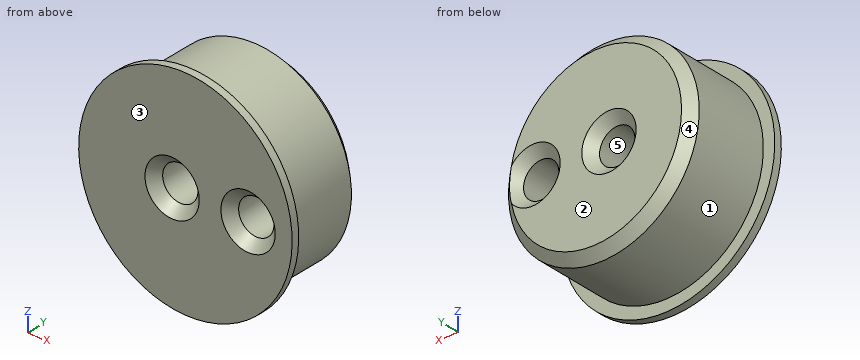
```python
from build123d import *
from build123d.topology import SkipClean

# Parameters (mm, degrees)
SKETCH_1_R      = 5.02
SKETCH_1_R_2    = 0.93
EXTRUDE_1_DEPTH = 4.4
EXTRUDE_START   = 0.4
SKETCH_3_R      = 5.62
SKETCH_3_R_2    = 0.93
EXTRUDE_2_DEPTH = 0.4
CHAMFER_1_SIZE  = 0.5


with BuildPart() as part:
    # 草图1 → 凸台-拉伸1 (new body)
    with BuildSketch(Plane(origin=(0, 0, 0), x_dir=(1, 0, 0), z_dir=(0, 1, 0))):
        with Locations(Location((0, 0, 0), (0, 0, 270))):
            Circle(SKETCH_1_R)
        with Locations(Location((3.3, 0, 0), (0, 0, 270))):
            Circle(SKETCH_1_R_2, mode=Mode.SUBTRACT)
        with Locations(Location((-0.7, 0, 0), (0, 0, 90))):
            Circle(SKETCH_1_R_2, mode=Mode.SUBTRACT)
    extrude(amount=EXTRUDE_1_DEPTH)

    # 草图3 → 凸台-拉伸2 (add)
    with SkipClean():  # the faces are left unmerged after this step: merging them gives an invalid solid
        with BuildSketch(Plane.XZ.offset(EXTRUDE_START)):
            with Locations(Location((0, 0, 0), (0, 0, 270))):
                Circle(SKETCH_3_R)
            with Locations(Location((3.3, 0, 0), (0, 0, 270))):
                Circle(SKETCH_3_R_2, mode=Mode.SUBTRACT)
            with Locations(Location((-0.7, 0, 0), (0, 0, 270))):
                Circle(SKETCH_3_R_2, mode=Mode.SUBTRACT)
        extrude(amount=-EXTRUDE_2_DEPTH)

    # 倒角1
    # the kernel refuses this chamfer: 0.5 mm, written as the material it takes off along each edge
    with BuildSketch(Plane(origin=(3.3, -0.4, 0), x_dir=(0, 0, -1), z_dir=(-1, 0, 0))) as chamfer_1_piece_1:
        Polygon((0.93 + CHAMFER_1_SIZE, 0), (0.93, -CHAMFER_1_SIZE), (0.93, 0), align=None)
    revolve(axis=Axis((3.3, -0.4, 0), (0, -1, 0)), mode=Mode.SUBTRACT)
    with BuildSketch(Plane(origin=(-0.7, -0.4, 0), x_dir=(0, 0, -1), z_dir=(-1, 0, 0))) as chamfer_1_piece_2:
        Polygon((0.93 + CHAMFER_1_SIZE, 0), (0.93, -CHAMFER_1_SIZE), (0.93, 0), align=None)
    revolve(axis=Axis((-0.7, -0.4, 0), (0, -1, 0)), mode=Mode.SUBTRACT)
    with BuildSketch(Plane(origin=(0, 4.4, 0), x_dir=(0, 0, 1), z_dir=(-1, 0, 0))) as chamfer_1_piece_3:
        Polygon((5.02, -CHAMFER_1_SIZE), (5.02 - CHAMFER_1_SIZE, 0), (5.02, 0), align=None)
    revolve(axis=Axis((0, 4.4, 0), (0, 1, 0)), mode=Mode.SUBTRACT)
    with BuildSketch(Plane(origin=(3.3, 4.4, 0), x_dir=(0, 0, 1), z_dir=(-1, 0, 0))) as chamfer_1_piece_4:
        Polygon((0.93 + CHAMFER_1_SIZE, 0), (0.93, -CHAMFER_1_SIZE), (0.93, 0), align=None)
    revolve(axis=Axis((3.3, 4.4, 0), (0, 1, 0)), mode=Mode.SUBTRACT)
    with BuildSketch(Plane(origin=(-0.7, 4.4, 0), x_dir=(0, 0, -1), z_dir=(1, 0, 0))) as chamfer_1_piece_5:
        Polygon((0.93 + CHAMFER_1_SIZE, 0), (0.93, -CHAMFER_1_SIZE), (0.93, 0), align=None)
    revolve(axis=Axis((-0.7, 4.4, 0), (0, 1, 0)), mode=Mode.SUBTRACT)


solid = part.part
```
Design review of the part built by this model. Coordinates are the model's own, in mm. Face numbers are marked on the shaded views. A direction names the side the tool comes from. Coordinates: 2 decimals unless noted, no trailing zeros. Write each loop counter-clockwise with the first axis right and the second up, starting at its lowest first coordinate (ties: lowest second). Pieces come first, ordered by that corner, then holes. Notation, with made-up numbers: M 21.25,35.25 L 36.25,35.25 A23 cw 36.25,53.25 Z; hole C 27.5,10 d5. An arc over 180 degrees is marked long. Answer as a JSON object with one key per item and string values.
Item 1: Draft analysis for pull direction Z (two halves, no side actions). For the marked faces 3, 4 and 5, state which applies: pulls with the +Z half, pulls with the -Z half, needs draft (parallel to the pull), parting line crosses it, or undercut.
Outcome:
{"face 3": "needs draft", "face 4": "parting line crosses it", "face 5": "undercut"}
Item 2: Insertion check: pin 1 Ø2 at (x, z) = (3.3, 0) entering from +Y; pin 2 Ø1.1 at (x, z) = (-0.7, 0) entering from +Y. Each pin has a flat end and moves straight along its axis. Give the tip position at first contact, or say it passes through.
Outcome:
{"pin 1": "y = 3.97", "pin 2": "through"}
Item 3: Wall thickness on probe 1 along X at (y, z) = (2.65, 0); probe 2 along X at (y, z) = (2.35, 0.5); probe 3 along Z at (x, y) = (-0.7, 1.45): over which ranges is each line inside the solid? List them lowest first.
Outcome:
{"probe 1": "-5.02 to -1.63, 0.23 to 2.37, 4.23 to 5.02", "probe 2": "-5 to -1.48, 0.08 to 2.52, 4.08 to 5", "probe 3": "-4.97 to -0.93, 0.93 to 4.97"}
Item 4: Add section A-A, the plane z = 0. Give the boundary of the cut face in (x, y) (3 decimals), and give its area (3 significant figures).
Outcome:
{"outline": "M -5.62,-0.4 L -2.13,-0.4 L -1.63,0.1 L -1.63,3.9 L -2.13,4.4 L -4.52,4.4 L -5.02,3.9 L -5.02,0 L -5.62,0 Z; M 0.23,0.1 L 0.73,-0.4 L 1.87,-0.4 L 2.37,0.1 L 2.37,3.9 L 1.87,4.4 L 0.73,4.4 L 0.23,3.9 Z; M 4.23,0.1 L 4.73,-0.4 L 5.62,-0.4 L 5.62,0 L 5.02,0 L 5.02,3.9 L 4.625,4.295 L 4.23,3.9 Z", "area": "29.6 mm²"}
Item 5: Add section B-B, the plane y = 3.4. Give the boundary of the cut face in (x, z).
Outcome:
{"outline": "C 0,0 d10.04; hole C -0.7,0 d1.86; hole C 3.3,0 d1.86"}
Item 6: Machinability: for the marked faces 1 and 2, which of the approach directions +Z, -Z, +X, -X, +Y, -Y give a long, thin tool a straight path to every point of the face, cutting with its end or side? Answer none if there is none.
Outcome:
{"face 1": "+Y", "face 2": "+Z, -Z, +X, -X, +Y"}
